from build123d import *

# Parameters (mm, degrees)
SKETCH1_R           = 75
BOSS_EXTRUDE3_DEPTH = 10
SKETCH1_4_R         = 75
SKETCH1_4_R_2       = 66.925057636
BOSS_EXTRUDE4_DEPTH = 50
SKETCH3_W           = 19
SKETCH3_H           = 18
BOSS_EXTRUDE5_DEPTH = 65
SKETCH4_W           = 19
SKETCH4_H           = 18
BOSS_EXTRUDE6_DEPTH = 45
SKETCH5_R           = 2.25
CUT_EXTRUDE1_DEPTH  = 15
FILLET2_R           = 3


with BuildPart() as part:
    # Sketch1 → Boss-Extrude3 (new body)
    with BuildSketch(Plane(origin=(0, 0, 0), x_dir=(1, 0, 0), z_dir=(0, 1, 0))):
        with Locations(Location((0, 0, 0), (0, 0, 270))):
            Circle(SKETCH1_R)
    extrude(amount=BOSS_EXTRUDE3_DEPTH)

    # Sketch1_4 → Boss-Extrude4 (add)
    with BuildSketch(Plane(origin=(0, 0, 0), x_dir=(1, 0, 0), z_dir=(0, 1, 0))):
        with Locations(Location((0, 0, 0), (0, 0, 270))):
            Circle(SKETCH1_4_R)
        with Locations(Location((0, 0, 0), (0, 0, 270))):
            Circle(SKETCH1_4_R_2, mode=Mode.SUBTRACT)
    extrude(amount=BOSS_EXTRUDE4_DEPTH)

    # Sketch3 → Boss-Extrude5 (add)
    with BuildSketch(Plane(origin=(75, 50, 0), x_dir=(0, 0, -1), z_dir=(1, 0, 0))):
        with Locations((0, -25)):
            Rectangle(SKETCH3_W, SKETCH3_H)
    extrude(amount=-BOSS_EXTRUDE5_DEPTH)

    # Sketch4 → Boss-Extrude6 (add)
    with BuildSketch(Plane(origin=(-75, 50, 0), x_dir=(0, 0, 1), z_dir=(-1, 0, 0))):
        with Locations((0, -25)):
            Rectangle(SKETCH4_W, SKETCH4_H)
    extrude(amount=-BOSS_EXTRUDE6_DEPTH)

    # Sketch5 → Cut-Extrude1 (cut)
    with BuildSketch(Plane(origin=(0, 34, 0), x_dir=(1, 0, 0), z_dir=(0, 1, 0))):
        with Locations(Location((14, 5.130777808, 0), (0, 0, 270))):
            Circle(SKETCH5_R)
        with Locations(Location((14, -4.869222192, 0), (0, 0, 270))):
            Circle(SKETCH5_R)
        with Locations(Location((-34, 5.130777808, 0), (0, 0, 270))):
            Circle(SKETCH5_R)
        with Locations(Location((-34, -4.869222192, 0), (0, 0, 270))):
            Circle(SKETCH5_R)
    extrude(amount=-CUT_EXTRUDE1_DEPTH, mode=Mode.SUBTRACT)

    # Fillet2
    fillet2_edges = [part.edges().sort_by_distance(p)[0] for p in [
        (0, 50, -75),
    ]]
    fillet(fillet2_edges, radius=FILLET2_R)


solid = part.part
Design review of the part built by this model. Coordinates are the model's own, in mm. A direction names the side the tool comes from. Round coordinates to 2 decimals unless told otherwise and drop trailing zeros. Write each loop counter-clockwise with the first axis right and the second up, starting at its lowest first coordinate (ties: lowest second). Pieces come first, ordered by that corner, then holes. Notation, with made-up numbers: (65, 80) - (96, 80) arc R20 ccw to (96, 117) - close; hole circle Ø11 at (66, -16). An arc over 180 degrees is marked (long way). Return JSON: item names as keys, results as strings. Group by question number.
Item 1: Machinability: for faces 1 (the face through (-21, 50, 64)), 2 (the face through (39, 16, 0)), 3 (the face through (12, 26.6, -4.1)), which of the approach directions +Z, -Z, +X, -X, +Y, -Y give a long, thin tool a straight path to every point of the face, cutting with its end or side? Answer none if there is none.
Item 2: We need section C-C on y = 38. Write out the cut boundary in (x, z).
Item 3: The part is to be moulded in two halves that separate along Z. For faces 4 (the face through (14, 19, -5)), 5 (the face through (1, 0, -1)), 6 (the face through (-32.103, 26.605, 6.079)), 7 (the face through (-45.636, 23.171, -59.517)), say which applies: pulls with the +Z half, pulls with the -Z half, needs draft (parallel to the pull), parting line crosses it, or undercut.
Item 4: Insertion check: P1, Ø5, axis at x = -34, z = 4.5, coming from the +Y side; P2, Ø10, axis at x = -18, y = 10.5, coming from the +Z side; P3, Ø4, axis at y = 35.5, z = 15, coming from the -X side; P4, Ø2.5, axis at x = -34, z = -5.13, coming from the -Y side. Each pin has a flat end and moves straight along its axis. Give the tip position at first contact, or say it passes through.
Item 5: We need section B-B on x = 0. Write out the cut boundary in (y, z), and give its area (3 significant figures).
Item 6: For probe 1 along Z at (x, y) = (21, 25); probe 2 along Y at (x, z) = (-60.5, 4.5); probe 3 along Z at (x, y) = (48, 21), list the stretches that pass through material, from the lowest coordinate up. Write a range as [from, to].
Item 7: We need section A-A on y = 27.5. Write out the cut boundary in (x, z), and give its area (3 significant figures).
Model answer:
{
 "1": {"face 1": "+Z, -Z, +X, -X, +Y", "face 2": "none", "face 3": "+Y"},
 "2": {"outline": "circle Ø150 at (0, 0); hole circle Ø133.85 at (0, 0)"},
 "3": {"face 4": "undercut", "face 5": "needs draft", "face 6": "undercut", "face 7": "parting line crosses it"},
 "4": {"P1": "stops at y = 34", "P2": "stops at z = 73.86", "P3": "stops at x = -73.86", "P4": "stops at y = 0"},
 "5": {"outline": "(0, -75) - (47, -75) arc R3 ccw to (50, -72) - (50, -66.93) - (10, -66.93) - (10, 66.93) - (50, 66.93) - (50, 72) arc R3 ccw to (47, 75) - (0, 75) - close", "area": "2,140 mm²"},
 "6": {"probe 1": "z = [-72, -63.54], [-9.5, 9.5], [63.54, 72]", "probe 2": "y = [0, 10], [16, 34]", "probe 3": "z = [-57.63, -46.64], [-9.5, 9.5], [46.64, 57.63]"},
 "7": {"outline": "(-75, -9.5) - (-74.4, -9.5) arc R75 ccw to (74.4, -9.5) - (75, -9.5) - (75, 9.5) - (74.4, 9.5) arc R75 ccw to (-74.4, 9.5) - (-75, 9.5) - close; hole (-66.25, -9.5) arc R66.93 ccw to (66.25, -9.5) - (10, -9.5) - (10, 9.5) - (66.25, 9.5) arc R66.93 ccw to (-66.25, 9.5) - (-30, 9.5) - (-30, -9.5) - close; hole circle Ø4.5 at (-34, -5.13); hole circle Ø4.5 at (-34, 4.87); hole circle Ø4.5 at (14, -5.13); hole circle Ø4.5 at (14, 4.87)", "area": "5,320 mm²"}
}
